The model under review builds one solid part; all positions refer to its coordinate system, in mm. Coordinates: 2 decimals unless noted, no trailing zeros. Write each loop counter-clockwise with the first axis right and the second up, starting at its lowest first coordinate (ties: lowest second). Pieces come first, ordered by that corner, then holes. Notation, with made-up numbers: M 35.25,16 L 47.25,16 A16 ccw 47.25,45 Z; hole C 56.25,2.25 d11. An arc over 180 degrees is marked long. Answer as CSV lines item,"result". Start each with the question number.
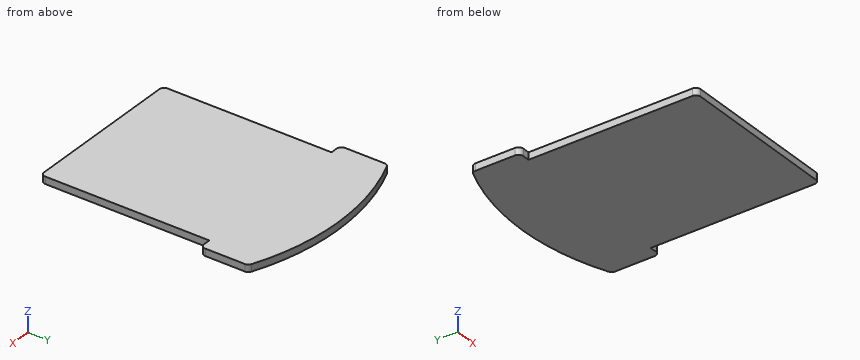
from build123d import *

# Parameters (mm, degrees)
ESQUISSE1_W        = 70
ESQUISSE1_H        = 71
BOSS_EXTRU_1_DEPTH = 3
BOSS_EXTRU_2_DEPTH = 3
CONG_1_R           = 2


with BuildPart() as part:
    # Esquisse1 → Boss.-Extru.1 (new body)
    with BuildSketch(Plane.XY):
        with Locations((35, 35.5)):
            Rectangle(ESQUISSE1_W, ESQUISSE1_H)
    extrude(amount=BOSS_EXTRU_1_DEPTH)

    # Esquisse2 → Boss.-Extru.2 (add)
    with BuildSketch(Plane.XY.offset(3)):
        with BuildLine():
            Line((-5, 91), (-5, 71))
            Line((-5, 71), (75, 71))
            Line((75, 71), (75, 91))
            ThreePointArc((75, 91), (35, 99.348486101), (-5, 91))
        make_face()
    extrude(amount=-BOSS_EXTRU_2_DEPTH)

    # Congé1
    cong_1_edges = [part.edges().sort_by_distance(p)[0] for p in [
        (-5, 91, 1.5),
        (75, 91, 1.5),
        (75, 71, 1.5),
        (-5, 71, 1.5),
        (70, 0, 1.5),
        (0, 0, 1.5),
    ]]
    fillet(cong_1_edges, radius=CONG_1_R)


solid = part.part
1) Take a section at A-A on z = 1.25. Give the boundary of the cut face in (x, y).
2) Take a section at B-B on y = 34.5. Give the boundary of the cut face in (x, z).
3) To check wall thickness, follow line 1 (X direction, y = 51, z = 1.4); line 2 (Y direction, x = 21.5, z = 1); line 3 (Y direction, x = 27, z = 0.9). State the ranges of each line that lie inside material, in increasing order. Write a range as [from, to].
4) Clearance check with flat-ended pins moving along their axes: pin 1 Ø0.9 at (y, z) = (20.5, 2) entering from -X; pin 2 Ø0.9 at (x, z) = (-1.5, 1.5) entering from -Y. State where each tip first meets the part, or that it passes through.
Results:
1,outline,"M -5,73 A2 ccw -3,71 L 0,71 L 0,2 A2 ccw 2,0 L 68,0 A2 ccw 70,2 L 70,71 L 73,71 A2 ccw 75,73 L 75,89.68 A2 ccw 73.78,91.52 A100 ccw -3.78,91.52 A2 ccw -5,89.68 Z"
2,outline,"M 0,0 L 70,0 L 70,3 L 0,3 Z"
3,line 1,"x = [0, 70]"
3,line 2,"y = [0, 98.43]"
3,line 3,"y = [0, 99.03]"
4,pin 1,"stops at x = 0"
4,pin 2,"stops at y = 71"
